Geometry check sheet. Reference: the model listing, model coordinates, mm. Give positions to 0.01 mm unless a question says otherwise; leave off trailing zeros. Order: outer loops, then holes, each group sorted by start corner. A loop starts at its lowest first (then second) coordinate and runs counter-clockwise, first axis right, second up. Notation, with made-up numbers: M 79.25,39.25 L 124.25,39.25 A27 cw 124.25,62.25 Z; hole C 42.25,-28 d7. An arc over 180 degrees is marked long. Put each result on its own line as item: value. Start each with the question number.
Q1. Mould release check, pull along Y, two halves, no side actions. Record for faces 1 (the cylindrical face through (51.02, 26.24, -37.57)), 2 (the cylindrical face through (338.767, 8.544, -37.567)), 3 (the cylindrical face through (381.438, 25.756, -65.028)), 4 (the flat face through (197, 0, -39)): +Y half, -Y half, draft (parallel to the pull), parting line (faces both ways), or undercut.
Q2. Section check C-C on x = 375. Record the cut outline in (y, z), then the cut area to 3 significant figures.
Q3. Material ranges on L1, parallel to Z at x = 25, y = 27; L2, parallel to X at y = 41, z = -57; L3, parallel to X at y = 17.5, z = -63, recorded low to high.
Q4. Section check B-B on z = -13. Record the cut outline in (x, y), then the cut area to 3 significant figures.
Q5. Section check A-A on y = 25.4. Record the cut outline in (x, z), then the cut area to 3 significant figures.
Q6. Section check D-D on x = 200. Record the cut outline in (y, z).
```python
from build123d import *

# Parameters (mm, degrees)
SKETCH1_W           = 400
SKETCH1_H           = 76.2
BOSS_EXTRUDE1_DEPTH = 50.8
SKETCH3_R           = 6.75
CUT_EXTRUDE2_DEPTH  = 50.8
SKETCH5_R           = 19
CUT_EXTRUDE3_DEPTH  = 77.2


with BuildPart() as part:
    # Sketch1 → Boss-Extrude1 (new body)
    with BuildSketch(Plane(origin=(0, 0, 0), x_dir=(1, 0, 0), z_dir=(0, 1, 0))):
        with Locations((200, 38.1)):
            Rectangle(SKETCH1_W, SKETCH1_H)
    extrude(amount=BOSS_EXTRUDE1_DEPTH)

    # Sketch3 → Cut-Extrude2 (cut)
    with BuildSketch(Plane(origin=(0, 50.8, 0), x_dir=(1, 0, 0), z_dir=(0, 1, 0))):
        with Locations((25, 63)):
            Circle(SKETCH3_R)
        with Locations((25, 13)):
            Circle(SKETCH3_R)
        with Locations((375, 63)):
            Circle(SKETCH3_R)
        with Locations((375, 13)):
            Circle(SKETCH3_R)
    extrude(amount=-CUT_EXTRUDE2_DEPTH, mode=Mode.SUBTRACT)

    # Sketch5 → Cut-Extrude3 (cut, through all)
    with BuildSketch(Plane.XY):
        with Locations((200, 25.4)):
            Circle(SKETCH5_R)
        with Locations((70, 25.4)):
            Circle(SKETCH5_R)
        with Locations((330, 25.4)):
            Circle(SKETCH5_R)
    extrude(amount=-CUT_EXTRUDE3_DEPTH, mode=Mode.SUBTRACT)


solid = part.part
```
Results found:
1. face 1: undercut
1. face 2: undercut
1. face 3: draft
1. face 4: -Y half
2. outline: M 0,-76.2 L 50.8,-76.2 L 50.8,-69.75 L 0,-69.75 Z; M 0,-56.25 L 50.8,-56.25 L 50.8,-19.75 L 0,-19.75 Z; M 0,-6.25 L 50.8,-6.25 L 50.8,0 L 0,0 Z
2. area: 2,500 mm^2
3. L1: z = -76.2 to -69.75, -56.25 to -19.75, -6.25 to 0
3. L2: x = 0 to 21.91, 28.09 to 59.15, 80.85 to 189.15, 210.85 to 319.15, 340.85 to 371.91, 378.09 to 400
3. L3: x = 0 to 18.25, 31.75 to 52.72, 87.28 to 182.72, 217.28 to 312.72, 347.28 to 368.25, 381.75 to 400
4. outline: M 0,0 L 18.25,0 L 18.25,50.8 L 0,50.8 Z; M 31.75,0 L 368.25,0 L 368.25,50.8 L 31.75,50.8 Z; M 381.75,0 L 400,0 L 400,50.8 L 381.75,50.8 Z; hole C 70,25.4 d38; hole C 200,25.4 d38; hole C 330,25.4 d38
4. area: 15,500 mm^2
5. outline: M 0,-76.2 L 51,-76.2 L 51,0 L 0,0 Z; M 89,-76.2 L 181,-76.2 L 181,0 L 89,0 Z; M 219,-76.2 L 311,-76.2 L 311,0 L 219,0 Z; M 349,-76.2 L 400,-76.2 L 400,0 L 349,0 Z; hole C 25,-63 d13.5; hole C 25,-13 d13.5; hole C 375,-63 d13.5; hole C 375,-13 d13.5
5. area: 21,200 mm^2
6. outline: M 0,-76.2 L 6.4,-76.2 L 6.4,0 L 0,0 Z; M 44.4,-76.2 L 50.8,-76.2 L 50.8,0 L 44.4,0 Z
